Autodesk Inventor part; units mm, degrees
ref_plane "YZ Plane" through (0, 0, 0) normal (1, 0, 0) x (0, 1, 0)
ref_plane "XZ Plane" through (0, 0, 0) normal (0, 1, 0) x (-1, 0, 0)
ref_plane "XY Plane" through (0, 0, 0) normal (0, 0, 1) x (1, 0, 0)
sketch "Sketch1" plane through (0, 0, 0) normal (0, 0, 1) x (1, 0, 0)
  line L0 (0, 0) -> (25, 0)
  line L1 (25, 0) -> (25, 40)
  line L2 (25, 40) -> (0, 40)
  line L3 (0, 40) -> (0, 0)
  dimension "d1" = 25
  dimension "d2" = 40
  dimension "d3" = 25
extrude "Extrusion1" add sketch "Sketch1" against normal blind 30
sketch "Sketch2" plane through (25, 0, 0) normal (1, 0, 0) x (0, 0, -1)
  line L0 (0, 0) -> (30, 0)
  circle A0 centre (15, 6.56) radius 2.46
extrude "Extrusion2" cut sketch "Sketch2" against normal blind 30
sketch "Sketch3" plane through (0, 0, 0) normal (-1, 0, 0) x (0, 0, 1)
  line L0 (0, 0) -> (-30, 0)
  line L1 (-25.05, 0) -> (-4.95, 0)
  line L2 (-4.95, 0) -> (-4.95, 33.12)
  line L3 (-4.95, 33.12) -> (-25.05, 33.12)
  line L4 (-25.05, 33.12) -> (-25.05, 0)
  dimension "d11" = 20.1
extrude "Extrusion3" cut sketch "Sketch3" against normal blind 20
sketch "Sketch4" plane through (0, 0, 0) normal (0, -1, 0) x (1, 0, 0)
  line L0 (20, -4.95) -> (20, -25.05)
  line L1 (20, -15) -> (25, -15)
  line L2 (25, 0) -> (25, -30)
  line L3 (20, -8.025) -> (25, -8.025)
  line L4 (25, -8.025) -> (25, -21.975)
  line L5 (25, -21.975) -> (20, -21.975)
  line L6 (20, -21.975) -> (20, -8.025)
  line L7 (20, -8.025) -> (25, -21.975) construction
  line L8 (25, -8.025) -> (20, -21.975) construction
  line L9 (25, -12.54) -> (25, -17.46)
  point P0 (0, 0)
  point P1 (22.5, -15)
  dimension "d14" = 13.95
extrude "Extrusion4" add sketch "Sketch4" along normal blind 15
sketch "Sketch5" plane through (20, 0, 0) normal (-1, 0, 0) x (0, 0, 1)
  circle A0 centre (-15, 6.56) radius 2.46
  circle A1 centre (-15, 6.56) radius 4.7025
  circle A2 centre (-15, 6.56) radius 2.46
  circle A3 centre (-15, 6.56) radius 2.46
  point P0 (0, 0)
  dimension "d17" = 9.405
extrude "Extrusion5" cut sketch "Sketch5" against normal blind 2.1
sketch "Sketch6" plane through (25, 0, 0) normal (1, 0, 0) x (0, 0, -1)
  circle A0 centre (15, 6.56) radius 4.7025
  line L0 (15, 6.56) -> (15, 23.56)
  circle A1 centre (15, 23.56) radius 2.46
  point P0 (0, 0)
  dimension "d20" = 17
  dimension "d21" = 4.92
extrude "Extrusion6" cut sketch "Sketch6" against normal blind 10 contours A1
sketch "Sketch7" plane through (20, 0, 0) normal (-1, 0, 0) x (0, 0, 1)
  circle A0 centre (-15, 23.56) radius 2.46
  circle A1 centre (-15, 23.56) radius 4.7025
  point P0 (0, 0)
  dimension "d24" = 9.405
extrude "Extrusion7" cut sketch "Sketch7" against normal blind 2.1
sketch "Sketch9" plane through (25, 0, 0) normal (1, 0, 0) x (0, 0, -1)
  circle A0 centre (15, 6.56) radius 2.46
  circle A1 centre (15, 6.56) radius 2.46
  circle A2 centre (15, 23.56) radius 2.46
  circle A3 centre (15, 23.56) radius 2.46
  line L0 (30, 40) -> (30, 0)
  line L1 (30, 0) -> (30, 40)
  line L2 (30, 40) -> (0, 40)
  line L3 (0, 40) -> (0, 0)
  line L4 (0, 0) -> (8.025, 0)
  line L5 (21.975, 0) -> (21.975, -15)
  line L6 (21.975, -15) -> (8.025, -15)
  line L7 (8.025, -15) -> (8.025, 0)
  line L8 (0, 0) -> (8.025, 0)
  line L9 (21.975, 0) -> (30, 0)
extrude "Extrusion8" add sketch "Sketch9" along normal blind 5
sketch "Sketch10" plane through (0, 40, 0) normal (0, 1, 0) x (1, 0, 0)
  line L0 (0, 30) -> (30, 30)
  line L1 (30, 0) -> (0, 0)
  line L2 (0, 30) -> (30, 30)
  line L3 (30, 30) -> (30, 0)
  line L4 (30, 0) -> (0, 0)
  line L5 (0, 0) -> (0, 30)
extrude "Extrusion9" add sketch "Sketch10" along normal blind 30
sketch "Sketch12" plane through (30, 0, 0) normal (1, 0, 0) x (0, 0, -1)
  circle A0 centre (15, 6.56) radius 2.46
  line L0 (15, 6.56) -> (15, 15.06)
  circle A1 centre (15, 15.06) radius 2.525
  point P0 (0, 0)
  dimension "d31" = 8.5
  dimension "d33" = 5.05
extrude "Extrusion10" cut sketch "Sketch12" against normal blind 30 contours A1
sketch "Sketch14" plane through (0, 0, 0) normal (0, 0, 1) x (1, 0, 0)
  line L0 (30, 70) -> (0, 70)
  line L1 (0, 70) -> (0, 85)
  line L2 (-15, 100) -> (-23, 100)
  line L3 (30, 0) -> (30, 70)
  line L4 (30, 109) -> (30, 70)
  arc A0 (0, 85) -> (-15, 100) centre (-15, 85) ccw
  line L5 (30, 105) -> (30, 100)
  line L6 (-23, 124) -> (15, 124)
  line L7 (-19, 122) -> (-23, 124)
  line L8 (-19, 122) -> (-15, 112)
  line L9 (-19, 102) -> (-23, 100)
  line L10 (-19, 102) -> (-15, 112)
  line L11 (30, 109) -> (15, 124)
  point P0 (0, 0)
  point P1 (0, 100)
  dimension "d47" = 30
  dimension "d54" = 15
extrude "Extrusion12" add sketch "Sketch14" against normal blind 30
sketch "Sketch15" plane through (0, 0, -25.05) normal (-1, 0, 0) x (0, 0, 1)
  line L0 (0, 33.12) -> (20.1, 33.12)
  line L1 (20.1, 33.12) -> (20.1, 0)
  line L2 (0, 33.12) -> (20.1, 33.12)
  line L3 (20.1, 33.12) -> (20.1, 31.1)
  line L4 (20.1, 31.1) -> (0, 31.1)
  line L5 (0, 31.1) -> (0, 33.12)
  point P0 (25.05, 0)
  dimension "d57" = 2.02
extrude "Extrusion13" add sketch "Sketch15" against normal blind 20
properties part number "20mm_x_30mm"
Verification items for the finished model (mm, model axes). A direction names the side the tool comes from. Coordinates: 2 decimals unless noted, no trailing zeros. Order: outer loops, then holes, each group sorted by start corner. A loop starts at its lowest first (then second) coordinate and runs counter-clockwise, first axis right, second up. Notation, with made-up numbers: (-18.75, 12) -> (18.25, 12) arc R29 ccw to (18.25, 43) -> close; hole circle Ø11 at (-39.5, 82.25). An arc over 180 degrees is marked (long way). Put each result on its own line as item: value. Start each with the question number.
1) Tool access check on faces 5 (the flat face through (10, 15, -4.95)), 6 (the cylindrical face through (21.035, 7.973, -10.515)), 7 (the flat face through (-19, 100, -15)), 8 (the flat face through (-21, 123, -15)). Record the directions out of +Z, -Z, +X, -X, +Y, -Y that give a thin tool (end or side, any length) a straight path to the whole face; none if there is none.
2) Cross-section at D-D (x = 5.5). Enter the section's corners in (y, z), plus the area to 3 significant figures.
3) Cross-section at B-B (y = 6.56). Enter the section's corners in (x, z), plus the area to 3 significant figures.
4) Cross-section at A-A (x = -17). Enter the section's corners in (y, z), plus the area to 3 significant figures.
5) Go/stop test with flat-tipped pins: pin 1 (12 mm diameter, centred on y = 85, z = -25, fed in from -X); pin 2 (9 mm diameter, centred on x = -18.5, z = -14, fed in from -Y); pin 3 (10.5 mm diameter, centred on y = 24.5, z = -13.5, fed in from -X); pin 4 (4 mm diameter, centred on y = 6.56, z = -15, fed in from +X). Record where each tip stops, or that it passes through.
6) Release check for a two-part mould opening along Y. For faces 1 (the flat face through (25, -7, -21.975)), 2 (the flat face through (18, 0, -27)), 3 (the flat face through (-21, 101, -15)), 4 (the flat face through (-4, 124, -15)) record: pulls with the +Y half, pulls with the -Y half, needs draft (parallel to the pull), parting line crosses it, or undercut.
7) Cross-section at C-C (z = -15). State how many separate pieces and enclosed holes the cut face has, plus the area to 3 significant figures.
8) Material ranges on L1, parallel to Z at x = 26.75, y = 23.56; L2, parallel to Y at x = 27.75, z = -15 (3 decimals); L3, parallel to X at y = 82.5, z = -6.5, recorded low to high.
Geometry check:
1. face 5: -X, -Y
1. face 6: -X
1. face 7: +Z, -Z, -X, -Y
1. face 8: +Z, -Z, -X
2. outline: (0, -30) -> (124, -30) -> (124, 0) -> (0, 0) -> (0, -4.95) -> (31.1, -4.95) -> (31.1, -25.05) -> (0, -25.05) -> close
2. area: 3,090 mm^2
3. outline: (0, -30) -> (30, -30) -> (30, -17.46) -> (22.1, -17.46) -> (22.1, -19.7) -> (20, -19.7) -> (20, -25.05) -> (0, -25.05) -> close; (0, -4.95) -> (20, -4.95) -> (20, -10.3) -> (22.1, -10.3) -> (22.1, -12.54) -> (30, -12.54) -> (30, 0) -> (0, 0) -> close
3. area: 439 mm^2
4. outline: (100, -30) -> (107, -30) -> (107, 0) -> (100, 0) -> close; (117, -30) -> (124, -30) -> (124, 0) -> (117, 0) -> close
4. area: 420 mm^2
5. pin 1: stops at x = -1.25
5. pin 2: stops at y = 99.97
5. pin 3: stops at x = 20
5. pin 4: passes through
6. face 1: needs draft
6. face 2: pulls with the -Y half
6. face 3: undercut
6. face 4: pulls with the +Y half
7. separate pieces: 4
7. enclosed holes: 0
7. area: 3,440 mm^2
8. L1: z = -30 to -17.46, -12.54 to 0
8. L2: y = -15 to 4.1, 9.02 to 12.535, 17.585 to 21.1, 26.02 to 111.25
8. L3: x = 0 to 30
